Autodesk Inventor part; units mm, degrees
ref_plane "工作平面1" through (0, 31, 0) normal (0, -1, 0) x (1, 0, 0)
ref_plane "YZ Plane" through (0, 0, 0) normal (1, 0, 0) x (0, 1, 0)
ref_plane "XZ Plane" through (0, 0, 0) normal (0, 1, 0) x (-1, 0, 0)
sketch "草圖1" plane through (0, 0, 0) normal (0, 1, 0) x (-1, 0, 0)
  circle A0 centre (0, 0) radius 2.45
  dimension "d0" = 4.9
extrude "擠出1" add sketch "草圖1" along normal blind 215
sketch "草圖2" plane through (0, 215, 0) normal (0, 1, 0) x (1, 0, 0)
  circle A0 centre (0, 0) radius 2.45
  circle A1 centre (0, 0) radius 2.3
  circle A2 centre (0, 0) radius 3.3
  dimension "d3" = 4.6
  dimension "d4" = 6.6
extrude "擠出2" add sketch "草圖2" along normal blind 3 contours A0 | A2
ref_plane "工作平面1" through (0, 31, 0) normal (0, -1, 0) x (1, 0, 0)
sketch "草圖3" plane through (0, 31, 0) normal (0, -1, 0) x (1, 0, 0)
  circle A0 centre (0, 0) radius 2.45
  circle A1 centre (0, 0) radius 3.25
  line L0 (3.25, 0) -> (-3.25, 0)
  line L1 (-3.25, 0) -> (-3.25, -12)
  line L2 (-3.25, -12) -> (3.25, -12)
  line L3 (3.25, -12) -> (3.25, 0)
  line L4 (1.6, -12) -> (-1.6, -12)
  line L5 (-1.6, -12) -> (-1.6, -7)
  line L6 (-1.6, -7) -> (1.6, -7)
  line L7 (1.6, -7) -> (1.6, -12)
  line L8 (1.5, -7) -> (-1.5, -7)
  line L9 (-1.5, -7) -> (-1.5, -10)
  line L10 (-1.5, -10) -> (1.5, -10)
  line L11 (1.5, -10) -> (1.5, -7)
  line L12 (1.5, -10) -> (1.2, -10)
  line L13 (1.2, -10) -> (1.6, -12)
  line L14 (-1.5, -10) -> (-1.2, -10)
  line L15 (-1.2, -10) -> (-1.6, -12)
  point P0 (0, -12)
  point P1 (0, -12)
  point P2 (0, -7)
  dimension "d17" = 6.5
  dimension "d9" = 12
  dimension "d11" = 5
  dimension "d12" = 3.2
  dimension "d13" = 3
  dimension "d14" = 3
  dimension "d15" = 0.3
  dimension "d16" = 0.3
  dimension "d18" = 6.5
extrude "擠出3" add sketch "草圖3" against normal blind 3 contours L0 A1 A0 | A0 L0 A1 | L3 L2 L7 L6 L5 L1 A1 | L13 L10 L11 L6 L7 | L5 L6 L9 L10 L15
pattern_linear "矩形陣列1" count 6 spacing 30 along (0, 1, 0) of "擠出3"
properties part number "[3DP]bar" material "MDF Medium Density Fiberboard"
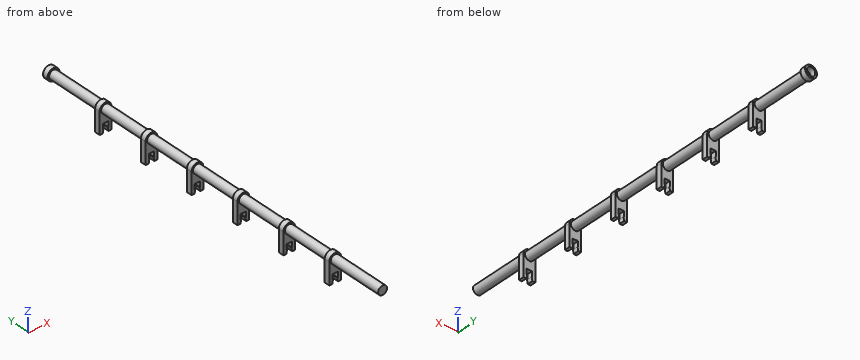
Source: CAD feature listing. Evaluate the final solid. Frame: model axes, mm. Give positions to 0.01 mm unless a question says otherwise; leave off trailing zeros. Write each loop counter-clockwise with the first axis right and the second up, starting at its lowest first coordinate (ties: lowest second). Pieces come first, ordered by that corner, then holes.
1. First-contact query: pin 1 (2 mm diameter, centred on x = -1, y = 29, fed in from -Z); pin 2 (3 mm diameter, centred on x = 2, z = -10, fed in from -Y); pin 3 (1.5 mm diameter, centred on x = 0, y = 152.5, fed in from -Z); pin 4 (4 mm diameter, centred on y = 28, z = -4.5, fed in from -X). Flat tips, straight axial feed; report the tip coordinate or a pass-through.
2. Section query A-A (y = 164). Return the cut outline in (x, z), then the cut area to 3 significant figures.
3. Material intervals for line 1 along Y through (x, z) = (-1.75, -4.5); line 2 along X through (y, z) = (215.9, 0), sorted ascending.
Output values:
1. pin 1: stops at z = -2.45
1. pin 2: stops at y = 31
1. pin 3: stops at z = -7
1. pin 4: passes through
2. outline: circle Ø4.9 at (0, 0)
2. area: 18.9 mm2
3. line 1: y = 31 to 34, 61 to 64, 91 to 94, 121 to 124, 151 to 154, 181 to 184
3. line 2: x = -3.3 to -2.3, 2.3 to 3.3
